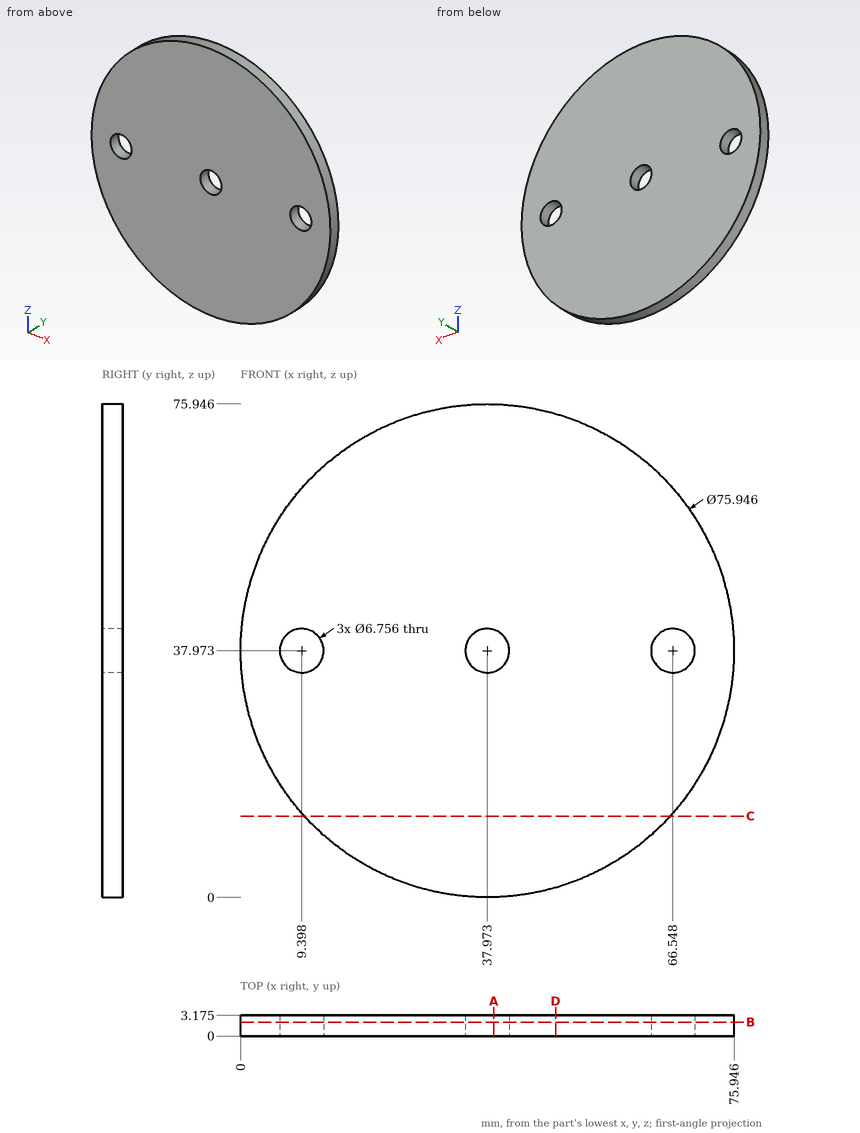
Part print with two shaded views. Sizes in mm from the minimum x, y, z corner. Round coordinates to 2 decimals unless told otherwise and drop trailing zeros. Order: outer loops, then holes, each group sorted by start corner. A loop starts at its lowest first (then second) coordinate and runs counter-clockwise, first axis right, second up. Notation, with made-up numbers: M 21.5,69 L 28.5,69 A21 ccw 28.5,98 Z; hole C 27.25,-36.75 d1. An arc over 180 degrees is marked long. Put each result on its own line as item: value. Start each with the question number.
1. Slice it at C-C on z = 12.5. List the corners of the cut face in (x, y) (1 decimal).
2. Slice it at D-D on x = 48.5. List the corners of the cut face in (y, z) (1 decimal).
3. Slice it at B-B on y = 2.15. List the corners of the cut face in (x, z) (1 decimal), then the cut area to 3 significant figures.
4. Drill centre lines: probe 1 along X at (y, z) = (1.1, 37); probe 2 along Z at (x, y) = (7.5, 2.45) (1 decimal); probe 3 along Z at (x, y) = (25, 0.8) (1 decimal). Where is each one in solid material? Low to high. Write a range as [from, to].
5. Drop flat-ended pins along their axis: pin 1 (5.5 mm diameter, centred on x = 66.548, z = 37.973, fed in from +Y); pin 2 (8 mm diameter, centred on x = 9.398, z = 37.973, fed in from +Y) (3 decimals); pin 3 (1.5 mm diameter, centred on y = 1, z = 14, fed in from +X). Give the stop position or say it passes through.
6. Slice it at A-A on x = 39. List the corners of the cut face in (y, z) (1 decimal).
Findings:
1. outline: M 9.8,0 L 66.1,0 L 66.1,3.2 L 9.8,3.2 Z
2. outline: M 0,1.5 L 3.2,1.5 L 3.2,74.5 L 0,74.5 Z
3. outline: C 38,38 d75.9; hole C 9.4,38 d6.8; hole C 38,38 d6.8; hole C 66.5,38 d6.8
3. area: 4,420 mm2
4. probe 1: [0.01, 6.16], [12.63, 34.74], [41.21, 63.31], [69.78, 75.93]
4. probe 2: [15.3, 35.2], [40.8, 60.6]
4. probe 3: [2.3, 73.7]
5. pin 1: through
5. pin 2: y = 3.175
5. pin 3: x = 68.02
6. outline: M 0,0 L 3.2,0 L 3.2,34.8 L 0,34.8 Z; M 0,41.2 L 3.2,41.2 L 3.2,75.9 L 0,75.9 Z
